For this review, use the dimensioned drawing (mm, ordinates from the lowest corner) and the shaded views. A direction names the side the tool comes from. Coordinates: 2 decimals unless noted, no trailing zeros. Write each loop counter-clockwise with the first axis right and the second up, starting at its lowest first coordinate (ties: lowest second). Pieces come first, ordered by that corner, then holes. Notation, with made-up numbers: (55.5, 45) -> (110.5, 45) arc R14 ccw to (110.5, 68) -> close; hole circle Ø11 at (-29, 37.5). An arc over 180 degrees is marked (long way). Put each result on its own line as item: value. Start each with the question number.
Item 1: Consider section A-A on y = 1.5. Give the boundary of the cut face in (x, z).
Item 2: The part is to be moulded in two halves that separate along Z. For the marked faces 1, 2 and 3, say which applies: +Z half, -Z half, draft (parallel to the pull), parting line (faces both ways), or undercut.
Item 3: To check wall thickness, follow L1, parallel to X at y = 2.5, z = 25; L2, parallel to X at y = 8.75, z = 46; L3, parallel to Z at x = 22.5, y = 8. State the ranges of each line that lie inside material, in increasing order.
Item 4: For the marked faces 4 and 5, list the 3-axis set-ups (+Z, -Z, +X, -X, +Y, -Y) from which the entire face can be reached by the end or side of a thin tool; tool diameter is ignored.
Item 5: Insertion check: P1, Ø19, axis at x = 25, z = 25, coming from the -Y side; P2, Ø9.5, axis at x = 50, z = 25, coming from the -Y side; P3, Ø3, axis at y = 10.5, z = 27, coming from the +X side; P4, Ø2, axis at x = 50, y = 14.5, coming from the -Z side. Each pin has a flat end and moves straight along its axis. Give the tip position at first contact, or say it passes through.
Item 6: Consider section B-B on x = 37.5. Give the boundary of the cut face in (y, z).
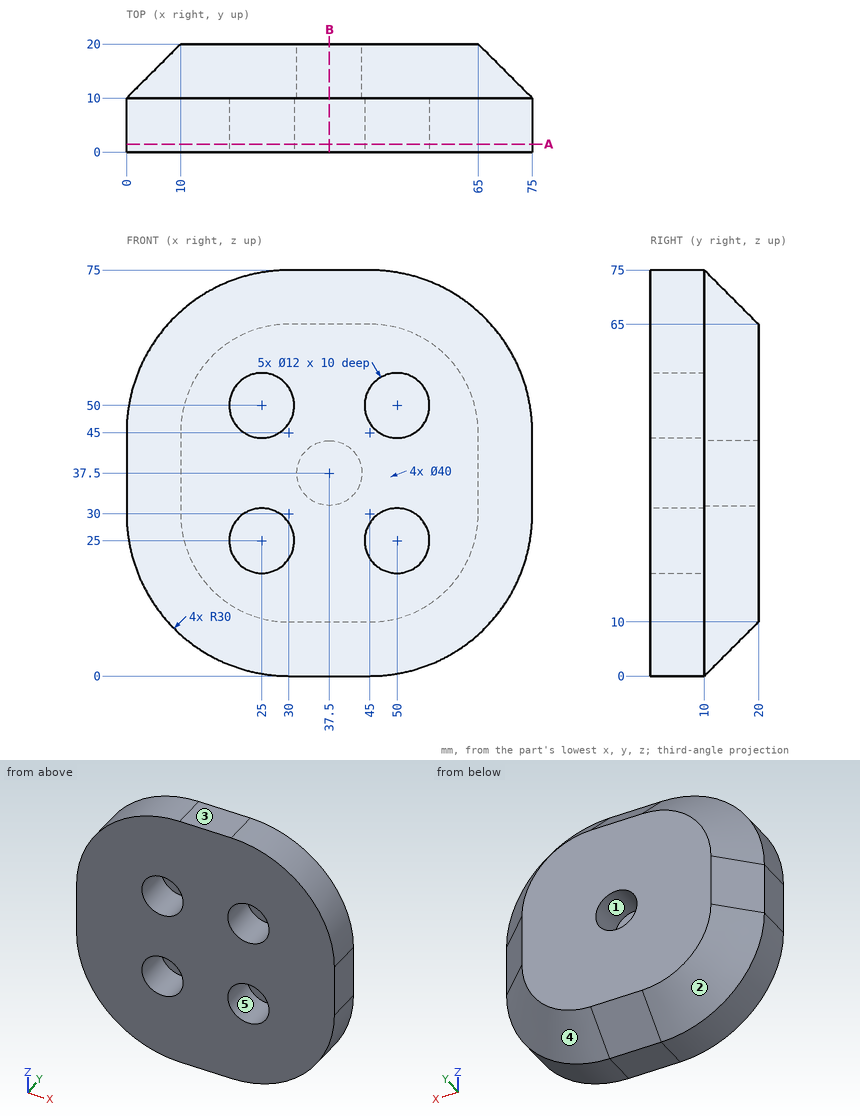
Return value:
1. outline: (0, 30) arc R30 ccw to (30, 0) -> (45, 0) arc R30 ccw to (75, 30) -> (75, 45) arc R30 ccw to (45, 75) -> (30, 75) arc R30 ccw to (0, 45) -> close; hole circle Ø12 at (25, 25); hole circle Ø12 at (25, 50); hole circle Ø12 at (50, 25); hole circle Ø12 at (50, 50)
2. face 1: undercut
2. face 2: -Z half
2. face 3: +Z half
3. L1: 0.42 to 19, 31 to 44, 56 to 74.58
3. L2: 0.02 to 20.53, 29.47 to 45.53, 54.47 to 74.98
3. L3: 0.95 to 19.55, 30.45 to 44.55, 55.45 to 74.05
4. face 4: -Z, +X, +Y
4. face 5: -Y
5. P1: y = 0
5. P2: y = 10
5. P3: x = 74.96
5. P4: z = 3.96
6. outline: (0, 0) -> (10, 0) -> (20, 10) -> (20, 31.5) -> (10, 31.5) -> (10, 43.5) -> (20, 43.5) -> (20, 65) -> (10, 75) -> (0, 75) -> close
